Input: part model. Units: mm. Frame: model coordinates. A direction names the side the tool comes from. Give positions to 0.01 mm unless a question says otherwise; leave off trailing zeros. Write each loop counter-clockwise with the first axis right and the second up, starting at its lowest first coordinate (ties: lowest second). Pieces come first, ordered by that corner, then holes. Notation, with made-up numbers: (81, 25) - (134, 25) arc R17 ccw to (134, 43) - close; hole circle Ø4 at (13, 89.25). An arc over 180 degrees is marked (long way). Answer as CSV lines item,"result".
```python
from build123d import *

# Parameters (mm, degrees)
BOSS_EXTRUDE1_DEPTH = 53
CUT_EXTRUDE1_DEPTH  = 52
FILLET1_R           = 1
FILLET3_R           = 1
SKETCH4_W           = 30
SKETCH4_H           = 200
CUT_EXTRUDE2_DEPTH  = 10


with BuildPart() as part:
    # Sketch2 → Boss-Extrude1 (new body)
    with BuildSketch(Plane.XY):
        Polygon((0, 0), (0, -4.14), (4.00969762, -1.825), (4.00969762, -14.175), (0, -11.86), (0, -19), (0, -219), (0, -226.14), (4.00969762, -223.825), (4.00969762, -236.175), (0, -233.86), (0, -238), (6, -238), (6, -233.86), (10.00969762, -236.175), (10.00969762, -223.825), (6, -226.14), (6, -11.86), (10.00969762, -14.175), (10.00969762, -1.825), (6, -4.14), (6, 0), align=None)
    extrude(amount=BOSS_EXTRUDE1_DEPTH)

    # Sketch3 → Cut-Extrude1 (cut)
    with BuildSketch(Plane(origin=(0, 0, 0), x_dir=(0, 0, -1), z_dir=(1, 0, 0))):
        Polygon((0, -119), (0, -58.5), (-2.8, -58.5), (-2.8, -179.5), (0, -179.5), align=None)
    extrude(amount=CUT_EXTRUDE1_DEPTH, mode=Mode.SUBTRACT)

    # Fillet1
    fillet1_edges = [part.edges().sort_by_distance(p)[0] for p in [
        (3, -179.5, 0),
        (3, -58.5, 0),
        (3, -58.5, 2.8),
        (0, -119, 2.8),
        (0, -58.5, 1.4),
        (3, -179.5, 2.8),
        (0, -179.5, 1.4),
    ]]
    fillet(fillet1_edges, radius=FILLET1_R)

    # Fillet3
    fillet3_edges = [part.edges().sort_by_distance(p)[0] for p in [
        (10.00969762, -1.825, 26.5),
        (10.00969762, -14.175, 26.5),
        (10.00969762, -223.825, 26.5),
        (10.00969762, -236.175, 26.5),
    ]]
    fillet(fillet3_edges, radius=FILLET3_R)

    # Sketch4 → Cut-Extrude2 (cut)
    with BuildSketch(Plane(origin=(6, 0, 0), x_dir=(0, 0, -1), z_dir=(1, 0, 0))):
        with Locations((-38, -119)):
            Rectangle(SKETCH4_W, SKETCH4_H)
    extrude(amount=-CUT_EXTRUDE2_DEPTH, mode=Mode.SUBTRACT)


solid = part.part
```
Item 1: Mould query, pull axis Y, two halves, no side actions, for faces 4 (the face through (10.01, -230, 26)), 5 (the face through (3, -19, 38)), 6 (the face through (3, 0, 26)). Classes: +Y half, -Y half, draft (parallel to the pull), parting line (faces both ways), or undercut.
The answers:
face 4,"draft"
face 5,"undercut"
face 6,"+Y half"
Item 2: Cut plane C-C on y = -190.5. Return the cut outline in (x, z).
The answers:
outline,"(0, 0) - (6, 0) - (6, 23) - (0, 23) - close"
Item 3: Cut plane B-B on z = 8.5. Return the cut outline in (x, y) (3 decimals).
The answers:
outline,"(0, -238) - (6, -238) - (6, -233.86) - (8.51, -235.309) arc R1 ccw to (10.01, -234.443) - (10.01, -225.557) arc R1 ccw to (8.51, -224.691) - (6, -226.14) - (6, -11.86) - (8.51, -13.309) arc R1 ccw to (10.01, -12.443) - (10.01, -3.557) arc R1 ccw to (8.51, -2.691) - (6, -4.14) - (6, 0) - (0, 0) - (0, -4.14) - (4.01, -1.825) - (4.01, -14.175) - (0, -11.86) - (0, -226.14) - (4.01, -223.825) - (4.01, -236.175) - (0, -233.86) - close"
Item 4: Reachability of faces 1 (the face through (3, -238, 26)), 2 (the face through (3, -120, 23)), 3 (the face through (4.01, -8, 26)) from +Z, -Z, +X, -X, +Y, -Y: full face, straight path, thin tool, end or side. Return the list, or none.
The answers:
face 1,"+Z, -Z, +X, -X, -Y"
face 2,"+Z, +X, -X"
face 3,"+Z, -Z"
Item 5: Ray query, line 1 (Y direction, x = 2.5, z = 38); line 2 (Y direction, x = 1, z = 35); line 3 (Y direction, x = 9, z = 51). Return the intervals inside material, ascending. Write a range as from..to.
The answers:
line 1,"-238..-235.3, -224.7..-219, -19..-13.3, -2.7..0"
line 2,"-238..-234.44, -225.56..-219, -19..-12.44, -3.56..0"
line 3,"-235.44..-224.56, -13.44..-2.56"
Item 6: Cut plane D-D on y = -152.5. Return the cut outline in (x, z).
The answers:
outline,"(0, 3.8) arc R1 ccw to (1, 2.8) - (6, 2.8) - (6, 23) - (0, 23) - close"
Item 7: Cut plane A-A on z = 46.5. Return the cut outline in (x, y) (3 decimals), plus the area to 3 significant figures.
The answers:
outline,"(0, -238) - (6, -238) - (6, -233.86) - (8.51, -235.309) arc R1 ccw to (10.01, -234.443) - (10.01, -225.557) arc R1 ccw to (8.51, -224.691) - (6, -226.14) - (6, -219) - (0, -219) - (0, -226.14) - (4.01, -223.825) - (4.01, -236.175) - (0, -233.86) - close; (0, -19) - (6, -19) - (6, -11.86) - (8.51, -13.309) arc R1 ccw to (10.01, -12.443) - (10.01, -3.557) arc R1 ccw to (8.51, -2.691) - (6, -4.14) - (6, 0) - (0, 0) - (0, -4.14) - (4.01, -1.825) - (4.01, -14.175) - (0, -11.86) - close"
area,"225 mm²"
Item 8: Contact query for flat-ended pins moving along their axis: pin 1 (1.5 mm diameter, centred on y = -105.5, z = 14, fed in from +X); pin 2 (13.5 mm diameter, centred on y = -5, z = 24.5, fed in from -X); pin 3 (5.5 mm diameter, centred on x = 3.5, y = -91, fed in from -Z); pin 4 (2 mm diameter, centred on y = -236, z = 38.5, fed in from +X). Output: stop coordinate, or through.
The answers:
pin 1,"x = 6"
pin 2,"x = 0"
pin 3,"z = 2.8"
pin 4,"x = 9.84"
